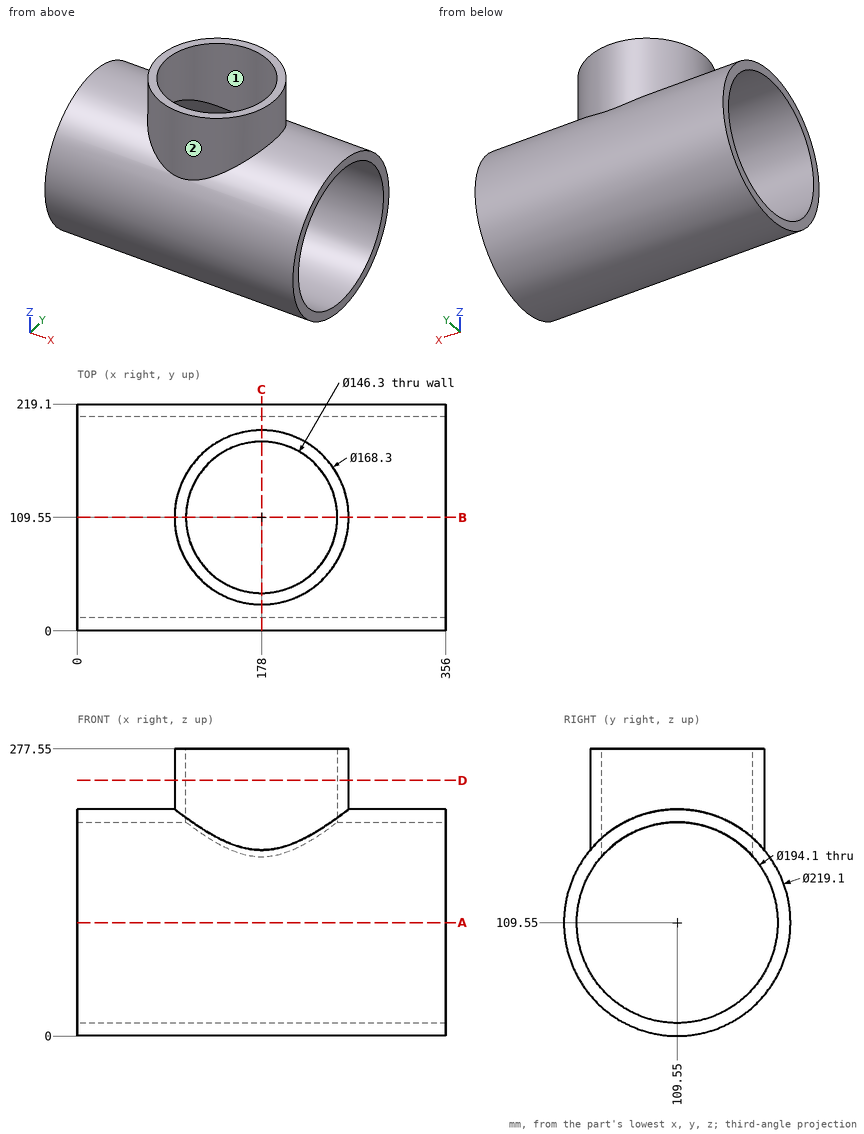
Part print with two shaded views. Sizes in mm from the minimum x, y, z corner. Coordinates: 2 decimals unless noted, no trailing zeros. Order: outer loops, then holes, each group sorted by start corner. A loop starts at its lowest first (then second) coordinate and runs counter-clockwise, first axis right, second up.
(1) Pin check, flat tips, straight feed: pin 1 Ø8 at (x, y) = (142.5, 160) entering from +Z; pin 2 Ø5 at (x, y) = (187, 159.5) entering from -Z; pin 3 Ø4 at (x, z) = (125, 158.5) entering from -Y. Stop position of each tip, or through.
Solution:
pin 1: stops at z = 29.21
pin 2: stops at z = 10.81
pin 3: stops at y = 10.57
(2) Mould opens along Y. For the marked faces 1 and 2 say: released by +Y, released by -Y, zero draft, split by the parting line, or undercut.
Solution:
face 1: undercut
face 2: split by the parting line
(3) Saw through at D-D, the plane z = 247. Write the cut outline in (x, y), and give its area (3 significant figures).
Solution:
outline: circle Ø168.3 at (178, 109.55); hole circle Ø146.3 at (178, 109.55)
area: 5,440 mm2
(4) Drill centre lines: L1, parallel to Y at x = 178, z = 204.5; L2, parallel to Y at x = 195, z = 110; L3, parallel to X at y = 147, z = 217.5. Where is each one in solid material? Low to high.
Solution:
L1: y = 25.4 to 36.4, 182.7 to 193.7
L2: y = 0 to 12.5, 206.6 to 219.1
L3: x = 102.64 to 115.16, 240.84 to 253.36
(5) Saw through at C-C, the plane x = 178. Write the cut outline in (y, z).
Solution:
outline: (25.4, 179.69) arc R109.55 ccw (long way) to (193.7, 179.69) - (193.7, 277.55) - (182.7, 277.55) - (182.7, 173.33) arc R97.05 cw (long way) to (36.4, 173.33) - (36.4, 277.55) - (25.4, 277.55) - close
(6) Saw through at B-B, the plane y = 109.55. Write the cut outline in (x, z), and give its area (3 significant figures).
Solution:
outline: (0, 0) - (356, 0) - (356, 12.5) - (0, 12.5) - close; (0, 206.6) - (104.85, 206.6) - (104.85, 277.55) - (93.85, 277.55) - (93.85, 219.1) - (0, 219.1) - close; (251.15, 206.6) - (356, 206.6) - (356, 219.1) - (262.15, 219.1) - (262.15, 277.55) - (251.15, 277.55) - close
area: 8,360 mm2
(7) Saw through at A-A, the plane z = 109.55. Write the cut outline in (x, y), and give its area (3 significant figures).
Solution:
outline: (0, 0) - (356, 0) - (356, 12.5) - (0, 12.5) - close; (0, 206.6) - (356, 206.6) - (356, 219.1) - (0, 219.1) - close
area: 8,900 mm2
